Source: CAD feature listing. Evaluate the final solid. Frame: model axes, mm. A direction names the side the tool comes from. Give positions to 0.01 mm unless a question says otherwise; leave off trailing zeros. Write each loop counter-clockwise with the first axis right and the second up, starting at its lowest first coordinate (ties: lowest second). Pieces come first, ordered by that corner, then holes. Notation, with made-up numbers: (-13, 64) -> (19, 64) arc R11 cw to (19, 80) -> close; hole circle Ø8 at (-12, -6.75). An arc over 180 degrees is marked (long way). Write item = value, one per line.
from build123d import *

# Parameters (mm, degrees)
SKETCH2_R               = 33.8
CUT_EXTRUDE1_DEPTH      = 19.1
CUT_EXTRUDE2_START      = -19.1
CUT_EXTRUDE2_DEPTH      = 2
CUT_EXTRUDE3_REACH      = 43.431
CUT_EXTRUDE3_END_RADIUS = 33.8
SKETCH6_R               = 1.6
CUT_EXTRUDE4_REACH      = 45.431
CUT_EXTRUDE4_START      = -2
SKETCH7_R               = 4.08
SKETCH8_R               = 9
CUT_EXTRUDE5_DEPTH      = 1.4
CUT_EXTRUDE6_REACH      = 43.024
CUT_EXTRUDE6_END_RADIUS = 33.8
SKETCH9_R               = 3.5
CUT_EXTRUDE8_REACH      = 44.024
CUT_EXTRUDE8_END_RADIUS = 33.8
SKETCH11_R              = 2
CUT_EXTRUDE9_REACH      = 44.024
CUT_EXTRUDE9_END_RADIUS = 33.8
CUT_EXTRUDE7_REACH      = 44.024
CUT_EXTRUDE7_END_RADIUS = 33.8
SKETCH10_R              = 1.45
BOSS_EXTRUDE1_DEPTH     = 3
CHAMFER1_SIZE           = 2


with BuildPart() as part:
    # Sketch1 → Revolve1 (revolve)
    with BuildSketch(Plane.XY, mode=Mode.PRIVATE) as revolve1_sk:
        with BuildLine():
            Line((0, -33.8), (0, 0))
            Line((0, 0), (33.8, 0))
            ThreePointArc((33.8, 0), (23.900209204, -23.900209204), (0, -33.8))
        make_face()
    revolve(revolve1_sk.sketch.rotate(Axis((0, -33.8, 0), (0, 1, 0)), 180), axis=Axis((0, -33.8, 0), (0, 1, 0)))

    # Sketch2 → Cut-Extrude1 (cut)
    with BuildSketch(Plane(origin=(0, 0, 0), x_dir=(1, 0, 0), z_dir=(0, 1, 0))):
        Circle(SKETCH2_R)
    extrude(amount=-CUT_EXTRUDE1_DEPTH, mode=Mode.SUBTRACT)

    # Sketch5 → Cut-Extrude2 (cut)
    with BuildSketch(Plane(origin=(0, 0, 0), x_dir=(1, 0, 0), z_dir=(0, 1, 0)).offset(CUT_EXTRUDE2_START)):
        with BuildLine():
            Line((-17.025732229, 6.571677263), (-23.544283672, 3.742739979))
            ThreePointArc((-23.544283672, 3.742739979), (-26, 0), (-23.544283672, -3.742739979))
            Line((-23.544283672, -3.742739979), (-17.025732229, -6.571677263))
            ThreePointArc((-17.025732229, -6.571677263), (0, -18.25), (17.025732229, -6.571677263))
            Line((17.025732229, -6.571677263), (23.544283672, -3.742739979))
            ThreePointArc((23.544283672, -3.742739979), (26, 0), (23.544283672, 3.742739979))
            Line((23.544283672, 3.742739979), (17.025732229, 6.571677263))
            ThreePointArc((17.025732229, 6.571677263), (0, 18.25), (-17.025732229, 6.571677263))
        make_face()
    extrude(amount=-CUT_EXTRUDE2_DEPTH, mode=Mode.SUBTRACT)

    # Cut-Extrude3: up to this sphere (the profile starts inside it)
    cut_extrude3_end = Location((0, 0, 0)) * Sphere(CUT_EXTRUDE3_END_RADIUS, mode=Mode.PRIVATE)
    # Sketch6 → Cut-Extrude3 (cut, up to the surface)
    with BuildSketch(Plane(origin=(0, -21.1, 0), x_dir=(1, 0, 0), z_dir=(0, 1, 0)), mode=Mode.PRIVATE) as cut_extrude3_sk1:
        with Locations(Location((-21.92, 0, 0), (0, 0, 270))):
            Circle(SKETCH6_R)
    cut_extrude3_tool1 = extrude(cut_extrude3_sk1.sketch, amount=-CUT_EXTRUDE3_REACH, mode=Mode.PRIVATE) & cut_extrude3_end
    add(cut_extrude3_tool1.solids().sort_by_distance((-21.92, -21.1, 0))[0], mode=Mode.SUBTRACT)
    # Sketch6 → Cut-Extrude3 (cut, up to the surface)
    with BuildSketch(Plane(origin=(0, -21.1, 0), x_dir=(1, 0, 0), z_dir=(0, 1, 0)), mode=Mode.PRIVATE) as cut_extrude3_sk2:
        with Locations(Location((21.92, 0, 0), (0, 0, 270))):
            Circle(SKETCH6_R)
    cut_extrude3_tool2 = extrude(cut_extrude3_sk2.sketch, amount=-CUT_EXTRUDE3_REACH, mode=Mode.PRIVATE) & cut_extrude3_end
    add(cut_extrude3_tool2.solids().sort_by_distance((21.92, -21.1, 0))[0], mode=Mode.SUBTRACT)

    # Sketch7 → Cut-Extrude4 (cut, up to next)
    with BuildSketch(Plane(origin=(0, -21.1, 0), x_dir=(1, 0, 0), z_dir=(0, 1, 0)).offset(CUT_EXTRUDE4_START), mode=Mode.PRIVATE) as cut_extrude4_sk1:
        with Locations((-21.92, 0)):
            Circle(SKETCH7_R)
    cut_extrude4_tool1 = extrude(cut_extrude4_sk1.sketch, amount=-CUT_EXTRUDE4_REACH, mode=Mode.PRIVATE) & part.part
    # Sketch7 → Cut-Extrude4 (cut, up to next)
    with BuildSketch(Plane(origin=(0, -21.1, 0), x_dir=(1, 0, 0), z_dir=(0, 1, 0)).offset(CUT_EXTRUDE4_START), mode=Mode.PRIVATE) as cut_extrude4_sk2:
        with Locations((21.92, 0)):
            Circle(SKETCH7_R)
    cut_extrude4_tool2 = extrude(cut_extrude4_sk2.sketch, amount=-CUT_EXTRUDE4_REACH, mode=Mode.PRIVATE) & part.part
    add(cut_extrude4_tool1.solids().sort_by_distance((-21.92, -23.1, 0))[0], mode=Mode.SUBTRACT)
    add(cut_extrude4_tool2.solids().sort_by_distance((21.92, -23.1, 0))[0], mode=Mode.SUBTRACT)

    # Sketch8 → Cut-Extrude5 (cut)
    with BuildSketch(Plane(origin=(0, -21.1, 0), x_dir=(1, 0, 0), z_dir=(0, 1, 0))):
        with Locations(Location((0, 0, 0), (0, 0, 270))):
            Circle(SKETCH8_R)
    extrude(amount=-CUT_EXTRUDE5_DEPTH, mode=Mode.SUBTRACT)

    # Cut-Extrude6: up to this sphere (the profile starts inside it)
    cut_extrude6_end = Location((0, 0, 0)) * Sphere(CUT_EXTRUDE6_END_RADIUS, mode=Mode.PRIVATE)
    # Sketch9 → Cut-Extrude6 (cut, up to the surface)
    with BuildSketch(Plane(origin=(0, -22.5, 0), x_dir=(1, 0, 0), z_dir=(0, 1, 0)), mode=Mode.PRIVATE) as cut_extrude6_sk1:
        with Locations(Location((0, 0, 0), (0, 0, 270))):
            Circle(SKETCH9_R)
    cut_extrude6_tool1 = extrude(cut_extrude6_sk1.sketch, amount=-CUT_EXTRUDE6_REACH, mode=Mode.PRIVATE) & cut_extrude6_end
    add(cut_extrude6_tool1.solids().sort_by_distance((0, -22.5, 0))[0], mode=Mode.SUBTRACT)

    # Cut-Extrude8: up to this sphere (the profile starts inside it)
    cut_extrude8_end = Location((0, 0, 0)) * Sphere(CUT_EXTRUDE8_END_RADIUS, mode=Mode.PRIVATE)
    # Sketch11 → Cut-Extrude8 (cut, up to the surface)
    with BuildSketch(Plane(origin=(0, -19.1, 0), x_dir=(1, 0, 0), z_dir=(0, 1, 0)), mode=Mode.PRIVATE) as cut_extrude8_sk1:
        with BuildLine():
            ThreePointArc((16.170155881, 15.717062664), (16.31818432, 12.8925118), (19.142735183, 13.040540238))
            Line((19.142735183, 13.040540238), (16.170155881, 15.717062664))
        make_face()
    cut_extrude8_tool1 = extrude(cut_extrude8_sk1.sketch, amount=-CUT_EXTRUDE8_REACH, mode=Mode.PRIVATE) & cut_extrude8_end
    add(cut_extrude8_tool1.solids().sort_by_distance((17.08847, -19.1, -13.748001))[0], mode=Mode.SUBTRACT)
    # Sketch11 → Cut-Extrude8 (cut, up to the surface)
    with BuildSketch(Plane(origin=(0, -19.1, 0), x_dir=(1, 0, 0), z_dir=(0, 1, 0)), mode=Mode.PRIVATE) as cut_extrude8_sk2:
        with BuildLine():
            Line((16.170155881, 15.717062664), (19.142735183, 13.040540238))
            ThreePointArc((19.142735183, 13.040540238), (19.523606385, 13.662065552), (19.656445532, 14.378801451))
            ThreePointArc((19.656445532, 14.378801451), (18.373181431, 16.245962304), (16.170155881, 15.717062664))
        make_face()
    cut_extrude8_tool2 = extrude(cut_extrude8_sk2.sketch, amount=-CUT_EXTRUDE8_REACH, mode=Mode.PRIVATE) & cut_extrude8_end
    add(cut_extrude8_tool2.solids().sort_by_distance((18.224421, -19.1, -15.009602))[0], mode=Mode.SUBTRACT)
    # Sketch11 → Cut-Extrude8 (cut, up to the surface)
    with BuildSketch(Plane(origin=(0, -19.1, 0), x_dir=(1, 0, 0), z_dir=(0, 1, 0)), mode=Mode.PRIVATE) as cut_extrude8_sk3:
        with Locations((17.656445532, 14.378801451)):
            Circle(SKETCH11_R)
    cut_extrude8_tool3 = extrude(cut_extrude8_sk3.sketch, amount=-CUT_EXTRUDE8_REACH, mode=Mode.PRIVATE) & cut_extrude8_end
    add(cut_extrude8_tool3.solids().sort_by_distance((17.656446, -19.1, -14.378801))[0], mode=Mode.SUBTRACT)
    # Sketch11 → Cut-Extrude8 (cut, up to the surface)
    with BuildSketch(Plane(origin=(0, -19.1, 0), x_dir=(1, 0, 0), z_dir=(0, 1, 0)), mode=Mode.PRIVATE) as cut_extrude8_sk4:
        Polygon((25.087893787, 7.687495387), (5.022983499, 25.754021759), (2.346461074, 22.781442457), (22.411371362, 4.714916085), align=None)
    cut_extrude8_tool4 = extrude(cut_extrude8_sk4.sketch, amount=-CUT_EXTRUDE8_REACH, mode=Mode.PRIVATE) & cut_extrude8_end
    add(cut_extrude8_tool4.solids().sort_by_distance((13.717177, -19.1, -15.234469))[0], mode=Mode.SUBTRACT)
    # Sketch11 → Cut-Extrude8 (cut, up to the surface)
    with BuildSketch(Plane(origin=(0, -19.1, 0), x_dir=(1, 0, 0), z_dir=(0, 1, 0)), mode=Mode.PRIVATE) as cut_extrude8_sk5:
        with BuildLine():
            ThreePointArc((16.170155881, 15.717062664), (16.31818432, 12.8925118), (19.142735183, 13.040540238))
            Line((19.142735183, 13.040540238), (16.170155881, 15.717062664))
        make_face()
    cut_extrude8_tool5 = extrude(cut_extrude8_sk5.sketch, amount=-CUT_EXTRUDE8_REACH, mode=Mode.PRIVATE) & cut_extrude8_end
    add(cut_extrude8_tool5.solids().sort_by_distance((17.08847, -19.1, -13.748001))[0], mode=Mode.SUBTRACT)
    # Sketch11 → Cut-Extrude8 (cut, up to the surface)
    with BuildSketch(Plane(origin=(0, -19.1, 0), x_dir=(1, 0, 0), z_dir=(0, 1, 0)), mode=Mode.PRIVATE) as cut_extrude8_sk6:
        with BuildLine():
            Line((16.170155881, 15.717062664), (19.142735183, 13.040540238))
            ThreePointArc((19.142735183, 13.040540238), (19.523606385, 13.662065552), (19.656445532, 14.378801451))
            ThreePointArc((19.656445532, 14.378801451), (18.373181431, 16.245962304), (16.170155881, 15.717062664))
        make_face()
    cut_extrude8_tool6 = extrude(cut_extrude8_sk6.sketch, amount=-CUT_EXTRUDE8_REACH, mode=Mode.PRIVATE) & cut_extrude8_end
    add(cut_extrude8_tool6.solids().sort_by_distance((18.224421, -19.1, -15.009602))[0], mode=Mode.SUBTRACT)

    # Cut-Extrude9: up to this sphere (the profile starts inside it)
    cut_extrude9_end = Location((0, 0, 0)) * Sphere(CUT_EXTRUDE9_END_RADIUS, mode=Mode.PRIVATE)
    # Sketch13 → Cut-Extrude9 (cut, up to the surface)
    with BuildSketch(Plane(origin=(0, -19.1, 0), x_dir=(1, 0, 0), z_dir=(0, 1, 0)), mode=Mode.PRIVATE) as cut_extrude9_sk1:
        Polygon((10.556374993, -19.224020053), (13.210464636, -21.224020053), (17.724077309, -15.234253728), (16.925441799, -14.632438705), (18.730886869, -12.236532175), (19.529522379, -12.838347198), (24.043135053, -6.848580873), (21.389045409, -4.848580873), align=None)
    cut_extrude9_tool1 = extrude(cut_extrude9_sk1.sketch, amount=-CUT_EXTRUDE9_REACH, mode=Mode.PRIVATE) & cut_extrude9_end
    add(cut_extrude9_tool1.solids().sort_by_distance((17.250772, -19.1, 12.999389))[0], mode=Mode.SUBTRACT)

    # Cut-Extrude7: up to this sphere (the profile starts inside it)
    cut_extrude7_end = Location((0, 0, 0)) * Sphere(CUT_EXTRUDE7_END_RADIUS, mode=Mode.PRIVATE)
    # Sketch10 → Cut-Extrude7 (cut, up to the surface)
    with BuildSketch(Plane(origin=(0, -19.1, 0), x_dir=(1, 0, 0), z_dir=(0, 1, 0)), mode=Mode.PRIVATE) as cut_extrude7_sk1:
        with Locations(Location((-16.069690242, -19.151111078, 0), (0, 0, 270))):
            Circle(SKETCH10_R)
    cut_extrude7_tool1 = extrude(cut_extrude7_sk1.sketch, amount=-CUT_EXTRUDE7_REACH, mode=Mode.PRIVATE) & cut_extrude7_end
    add(cut_extrude7_tool1.solids().sort_by_distance((-16.06969, -19.1, 19.151111))[0], mode=Mode.SUBTRACT)
    # Sketch10 → Cut-Extrude7 (cut, up to the surface)
    with BuildSketch(Plane(origin=(0, -19.1, 0), x_dir=(1, 0, 0), z_dir=(0, 1, 0)), mode=Mode.PRIVATE) as cut_extrude7_sk2:
        with Locations(Location((16.069690242, 19.151111078, 0), (0, 0, 270))):
            Circle(SKETCH10_R)
    cut_extrude7_tool2 = extrude(cut_extrude7_sk2.sketch, amount=-CUT_EXTRUDE7_REACH, mode=Mode.PRIVATE) & cut_extrude7_end
    add(cut_extrude7_tool2.solids().sort_by_distance((16.06969, -19.1, -19.151111))[0], mode=Mode.SUBTRACT)

    # Sketch14 → Boss-Extrude1 (add)
    with BuildSketch(Plane(origin=(0, -19.1, 0), x_dir=(1, 0, 0), z_dir=(0, 1, 0))):
        Polygon((-5.819186048, 18.818103207), (2.060921488, 24.97471796), (2.676582963, 24.186707207), (-5.203524573, 18.030092453), align=None)
        Polygon((-23.943433381, 4.657889274), (-16.063325845, 10.814504028), (-15.44766437, 10.026493274), (-23.327771906, 3.869878521), align=None)
    extrude(amount=BOSS_EXTRUDE1_DEPTH)

    # Chamfer1
    # the kernel refuses this chamfer: 2 mm, written as the material it takes off along each edge
    with BuildSketch(Plane(origin=(-21.92, -23.1, 0), x_dir=(0, 0, 1), z_dir=(-1, 0, 0))) as chamfer1_piece_1:
        Polygon((1.6 + CHAMFER1_SIZE, 0), (1.6, CHAMFER1_SIZE), (1.6, 0), align=None)
    revolve(axis=Axis((-21.92, -23.1, 0), (0, 1, 0)), mode=Mode.SUBTRACT)
    with BuildSketch(Plane(origin=(21.92, -23.1, 0), x_dir=(0, 0, 1), z_dir=(-1, 0, 0))) as chamfer1_piece_2:
        Polygon((1.6 + CHAMFER1_SIZE, 0), (1.6, CHAMFER1_SIZE), (1.6, 0), align=None)
    revolve(axis=Axis((21.92, -23.1, 0), (0, 1, 0)), mode=Mode.SUBTRACT)


solid = part.part
1) Draft query along X for faces 4 (the flat face through (-1.21, -17.62, -21.15)), 5 (the flat face through (-1.6, -16.1, -21.5)), 6 (the flat face through (23.434, -21.299, -5.85)). Return one class per face: pulls with the +X half, pulls with the -X half, needs draft (parallel to the pull), parting line crosses it, or undercut.
Computed:
face_4 = pulls with the +X half
face_5 = needs draft
face_6 = undercut
2) Cut plane D-D (z = 0). Return the cut outline in (x, y), then the cut area to 3 significant figures.
Computed:
outline = (-27.89, -19.1) arc R33.8 ccw to (-25.08, -22.66) -> (-23.52, -21.1) -> (-26, -21.1) -> (-26, -19.1) -> close; (-20.32, -21.1) -> (-18.32, -23.1) -> (-17.84, -23.1) -> (-17.84, -28.71) arc R33.8 ccw to (-3.5, -33.62) -> (-3.5, -22.5) -> (-9, -22.5) -> (-9, -21.1) -> close; (3.5, -33.62) arc R33.8 ccw to (17.84, -28.71) -> (17.84, -23.1) -> (18.32, -23.1) -> (20.32, -21.1) -> (9, -21.1) -> (9, -22.5) -> (3.5, -22.5) -> close; (23.52, -21.1) -> (25.08, -22.66) arc R33.8 ccw to (27.89, -19.1) -> (26, -19.1) -> (26, -21.1) -> close
area = 306 mm²
3) Material intervals for L1, parallel to X at y = -26.35, z = 0; L2, parallel to X at y = -19.5, z = -9; L3, parallel to Z at x = 8, y = -20, sorted ascending.
Computed:
L1 = -17.84 to -3.5, 3.5 to 17.84
L2 = -26.1 to -15.88, 15.88 to 17.65, 23.63 to 26.1
L3 = -26.05 to -23.07, -17.69 to -16.4, 16.4 to 26.05
4) Cut plane B-B (x = 0). Return the cut outline in (y, z).
Computed:
outline = (-33.62, -3.5) arc R33.8 ccw to (-19.1, -27.89) -> (-19.1, -23.36) -> (-16.1, -23.36) -> (-16.1, -22.1) -> (-19.1, -22.1) -> (-19.1, -18.25) -> (-21.1, -18.25) -> (-21.1, -9) -> (-22.5, -9) -> (-22.5, -3.5) -> close; (-33.62, 3.5) -> (-22.5, 3.5) -> (-22.5, 9) -> (-21.1, 9) -> (-21.1, 18.25) -> (-19.1, 18.25) -> (-19.1, 27.89) arc R33.8 ccw to start
5) Contact query for flat-ended pins moving along their axis: pin 1 (10 mm diameter, centred on x = -20, y = -24, fed in from +Z); pin 2 (9.5 mm diameter, centred on x = -21.92, z = 0, fed in from -Y); pin 3 (5 mm diameter, centred on x = 2, y = -18.5, fed in from -Z); pin 4 (2.5 mm diameter, centred on x = 16.07, z = -19.15, fed in from -Y). Output: stop coordinate, or through.
Computed:
pin_1 = 21.3
pin_2 = -29.11
pin_3 = -27.89
pin_4 = through
6) Access query for faces 1 (the flat face through (11.865, -21.628, 20.21)), 2 (the conical face through (-20.017, -21.419, -0.25)), 3 (the flat face through (-20.239, -20.086, -5.177)). Directions: +Z, -Z, +X, -X, +Y, -Y. A direction counts if a zero-diameter tool reaches every point of the face in a straight line with its end or side. Return the directions, or none.
Computed:
face_1 = +Y, -Y
face_2 = -Y
face_3 = +Y
7) Cut plane A-A (y = -16.75). Return the cut outline in (x, z).
Computed:
outline = (-23.94, -4.66) -> (-16.06, -10.81) -> (-15.45, -10.03) -> (-23.33, -3.87) -> close; (-5.82, -18.82) -> (2.06, -24.97) -> (2.68, -24.19) -> (-5.2, -18.03) -> close
8) Cut plane C-C (z = -22). Return the cut outline in (x, y).
Computed:
outline = (-17.14, -19.1) arc R25.66 ccw to (3.21, -25.46) -> (3.21, -19.1) -> (-0.12, -19.1) -> (-0.12, -16.1) -> (-1.75, -16.1) -> (-1.75, -19.1) -> close; (9.19, -23.96) arc R25.66 ccw to (17.14, -19.1) -> (9.19, -19.1) -> close
